For this review, use the dimensioned drawing (mm, ordinates from the lowest corner) and the shaded views. A direction names the side the tool comes from. Coordinates: 2 decimals unless noted, no trailing zeros. Loops run counter-clockwise (first coordinate to the right, second up) from the corner with the lowest first, then second, coordinate; pieces in that order, holes last. Notation, with made-up numbers: (-10.5, -2.5) - (1.5, -2.5) arc R16 cw to (1.5, 24.5) - close; hole circle Ø7 at (-34.5, 39). An arc over 180 degrees is marked (long way). Answer in a Markdown table with one row per item. Add a question column.
(1) We need section B-B on y = 32. Write out the cut boundary in (x, z).
(2) We need section C-C on z = 16.5. Write out the cut boundary in (x, y).
(3) We need section D-D on x = 4.5. Write out the cut boundary in (y, z) (1 decimal).
(4) We need section A-A on x = 20. Write out the cut boundary in (y, z).
(5) For P1, Ø1, axis at y = 40.5, z = 16.5, coming from the -X side; P2, Ø0.6, axis at y = 40, z = 18.5, coming from the +X side; P3, Ø12, axis at x = 10.5, z = 14.5, coming from the -Y side, all flat-tipped, find the tip position at first contact; note any pin that passes through.
(6) For line 1 along Y through (x, z) = (35, 45.4); line 2 along Y through (x, z) = (35, 45.85); line 3 along Z through (x, y) = (21, 15.5), list the stretches that pass through material, from the lowest coordinate up.
(7) Machinability: for the marked faces 1 and 2, which of the approach directions +Z, -Z, +X, -X, +Y, -Y give a long, thin tool a straight path to every point of the face, cutting with its end or side? Answer none if there is none.
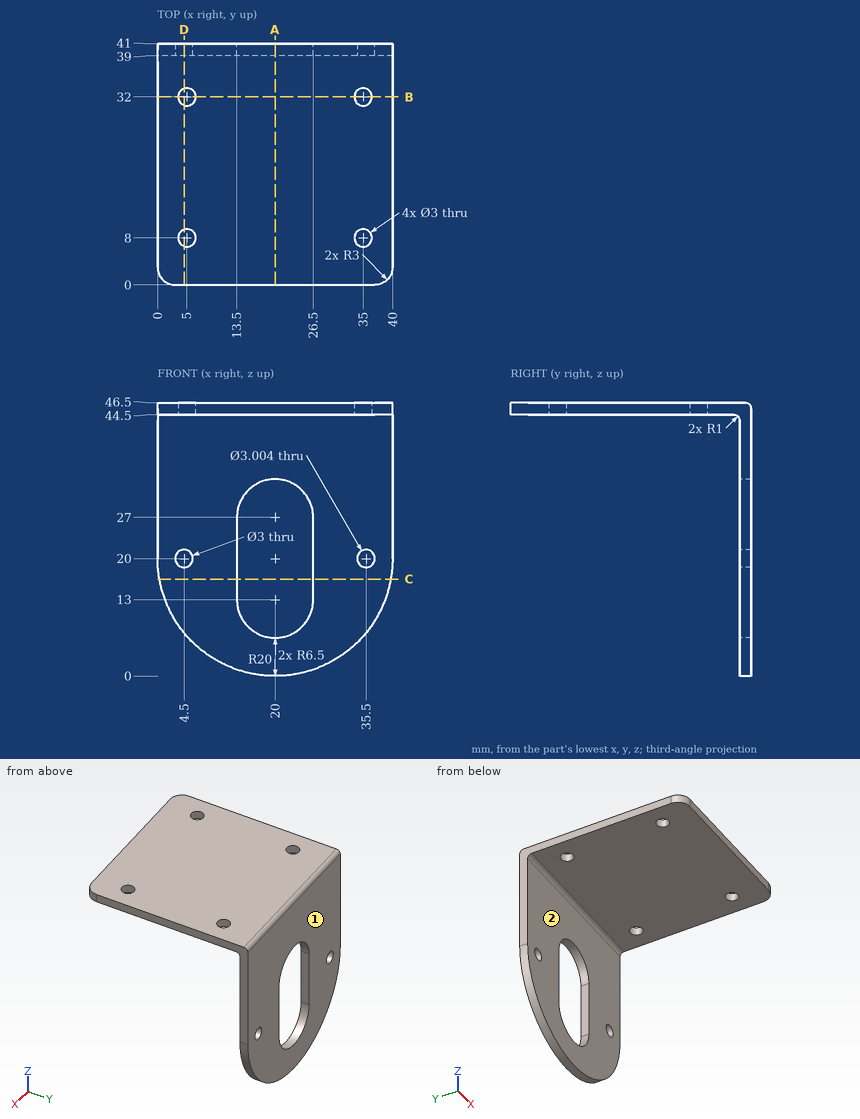
Outcome:
| question | item | result |
|---|---|---|
| 1 | outline | (0, 44.5) - (3.5, 44.5) - (3.5, 46.5) - (0, 46.5) - close; (6.5, 44.5) - (33.5, 44.5) - (33.5, 46.5) - (6.5, 46.5) - close; (36.5, 44.5) - (40, 44.5) - (40, 46.5) - (36.5, 46.5) - close |
| 2 | outline | (0.31, 39) - (13.5, 39) - (13.5, 41) - (0.31, 41) - close; (26.5, 39) - (39.69, 39) - (39.69, 41) - (26.5, 41) - close |
| 3 | outline | (0, 44.5) - (6.6, 44.5) - (6.6, 46.5) - (0, 46.5) - close; (9.4, 44.5) - (30.6, 44.5) - (30.6, 46.5) - (9.4, 46.5) - close; (33.4, 44.5) - (38, 44.5) arc R1 cw to (39, 43.5) - (39, 21.5) - (41, 21.5) - (41, 45.5) arc R1 ccw to (40, 46.5) - (33.4, 46.5) - close; (39, 7.4) - (41, 7.4) - (41, 18.5) - (39, 18.5) - close |
| 4 | outline | (0, 44.5) - (38, 44.5) arc R1 cw to (39, 43.5) - (39, 33.5) - (41, 33.5) - (41, 45.5) arc R1 ccw to (40, 46.5) - (0, 46.5) - close; (39, 0) - (41, 0) - (41, 6.5) - (39, 6.5) - close |
| 5 | P1 | x = 0.23 |
| 5 | P2 | x = 39.96 |
| 5 | P3 | y = 39 |
| 6 | line 1 | 0 to 6.5, 9.5 to 30.5, 33.5 to 41 |
| 6 | line 2 | 0 to 6.5, 9.5 to 30.5, 33.5 to 40.94 |
| 6 | line 3 | 44.5 to 46.5 |
| 7 | face 1 | +Z, -Z, +X, -X, +Y |
| 7 | face 2 | -Z, +X, -X, -Y |
